Input: part model. Units: mm. Frame: model coordinates. Coordinates: 2 decimals unless noted, no trailing zeros. Order: outer loops, then holes, each group sorted by start corner. A loop starts at its lowest first (then second) coordinate and runs counter-clockwise, first axis right, second up. Notation, with made-up numbers: (-38.5, -39.75) - (14.5, -39.75) arc R21 cw to (14.5, -30.75) - close; hole circle Ø3 at (74.25, 16.5). An arc over 180 degrees is marked (long way). One line per question, with ' | ' between items. Start each with the question number.
Autodesk Inventor part; units mm, degrees
ref_plane "Work Plane1" through (0, -15, 0) normal (0, 1, 0) x (-1, 0, 0)
ref_plane "YZ Plane" through (0, 0, 0) normal (1, 0, 0) x (0, 1, 0)
ref_plane "XY Plane" through (0, 0, 0) normal (0, 0, 1) x (1, 0, 0)
sketch "Sketch1" plane through (0, 0, 0) normal (0, 0, 1) x (1, 0, 0)
  arc A0 (0, -19.8) -> (0, 19.8) centre (0, 0) ccw
  line L0 (0, 19.8) -> (0, -19.8)
  dimension "d0" = 19.8
revolve "Revolution1" add sketch "Sketch1" angle 360 about axis through (0, 19.8, 0) along (0, -1, 0)
ref_plane "Work Plane1" through (0, -15, 0) normal (0, 1, 0) x (-1, 0, 0)
split_face "Split1"
split "Split2" plane through (0, -15, 0) removes the side toward (0, -1, 0)
sketch "Sketch3" plane through (0, -15, 0) normal (0, 1, 0) x (-1, 0, 0)
  line L0 (-7.5, -7.5) -> (7.5, -7.5)
  line L1 (7.5, -7.5) -> (7.5, 7.5)
  line L2 (7.5, 7.5) -> (-7.5, 7.5)
  line L3 (-7.5, 7.5) -> (-7.5, -7.5)
  line L4 (-7.5, -7.5) -> (7.5, 7.5) construction
  line L5 (7.5, -7.5) -> (-7.5, 7.5) construction
  point P0 (0, 0)
  dimension "d10" = 15
  dimension "d11" = 15
extrude "Extrusion1" cut sketch "Sketch3" along normal blind 20
properties part number "Femoral Head DP-2" material "Silver"
(1) Pin query (flat end, axial travel): pin 1 (16.5 mm diameter, centred on x = -2.5, y = -1, fed in from -Z); pin 2 (16.5 mm diameter, centred on x = 2.5, y = -6, fed in from +Z); pin 3 (5 mm diameter, centred on y = 3.5, z = -10, fed in from +X). Return the tip coordinate at first contact, or that it passes through.
(2) Section C-C (z = -1). Output: boundary loops of the cut face in (x, y), then the cut area to 3 significant figures.
(3) Section A-A (y = -4). Output: boundary loops of the cut face in (x, z), then the cut area to 3 significant figures.
(4) Section D-D (y = 15). Output: boundary loops of the cut face in (x, z), then the cut area to 3 significant figures.
(5) Section B-B (x = -3). Output: boundary loops of the cut face in (y, z), then the cut area to 3 significant figures.
(6) Material intervals for line 1 along Z through (x, y) = (-5, -12.5); line 2 along X through (y, z) = (-1, 0); line 3 along X through (y, z) = (-6, 5), sorted ascending. Write a range as from..to.
(7) Draft query along Z for faces 1 (the face through (0, 5, 0)), 2 (the face through (8, -15, 0)), 3 (the face through (7.5, -5, 0)). Return one class per face: +Z half, -Z half, draft (parallel to the pull), parting line (faces both ways), or undercut.
Worked answers:
1) pin 1: stops at z = -19.8 | pin 2: stops at z = 19.8 | pin 3: stops at x = 18.07
2) outline: (-12.89, -15) - (-7.5, -15) - (-7.5, 5) - (7.5, 5) - (7.5, -15) - (12.89, -15) arc R19.77 ccw (long way) to start | area: 844 mm²
3) outline: circle Ø38.78 at (0, 0); hole (-7.5, -7.5) - (7.5, -7.5) - (7.5, 7.5) - (-7.5, 7.5) - close | area: 956 mm²
4) outline: circle Ø25.85 at (0, 0) | area: 525 mm²
5) outline: (-15, -12.57) arc R19.57 ccw (long way) to (-15, 12.57) - (-15, 7.5) - (5, 7.5) - (5, -7.5) - (-15, -7.5) - close | area: 825 mm²
6) line 1: z = -14.52..-7.5, 7.5..14.52 | line 2: x = -19.77..-7.5, 7.5..19.77 | line 3: x = -18.19..-7.5, 7.5..18.19
7) face 1: undercut | face 2: draft | face 3: undercut
